Part print with two shaded views. Sizes in mm from the minimum x, y, z corner. Coordinates: 2 decimals unless noted, no trailing zeros. Write each loop counter-clockwise with the first axis right and the second up, starting at its lowest first coordinate (ties: lowest second). Pieces come first, ordered by that corner, then holes. Notation, with made-up numbers: M -23.75,29.25 L 19.25,29.25 A21 ccw 19.25,41.25 Z; hole C 53.5,-27 d7. An arc over 180 degrees is marked long. One line per question, with ' | ' between items. Start each with the question number.
(1) Flat gauge pins, fed straight in: pin 1 Ø5 at (y, z) = (7, 8) entering from -X; pin 2 Ø4.5 at (x, y) = (17.5, 17.5) entering from -Z. Where does each tip first touch, or does it go through?
(2) Two-plate mould, pull along Y, no slides. Class the marked faces 1, 2 and 3: +Y half, -Y half, draft (parallel to the pull), parting line (faces both ways), or undercut.
(3) Cut at D-D (x = 12.5). Write the cut outline in (y, z).
(4) Wall check: probe 1 along Y at (x, z) = (17.5, 2.5); probe 2 along Z at (x, y) = (4.5, 10); probe 3 along X at (y, z) = (5, 9). Give the ranges that are in metal, low to high.
(5) Cut at B-B (z = 3.5). Write the cut outline in (x, y).
(6) Cut at A-A (x = 17.5). Write the cut outline in (y, z).
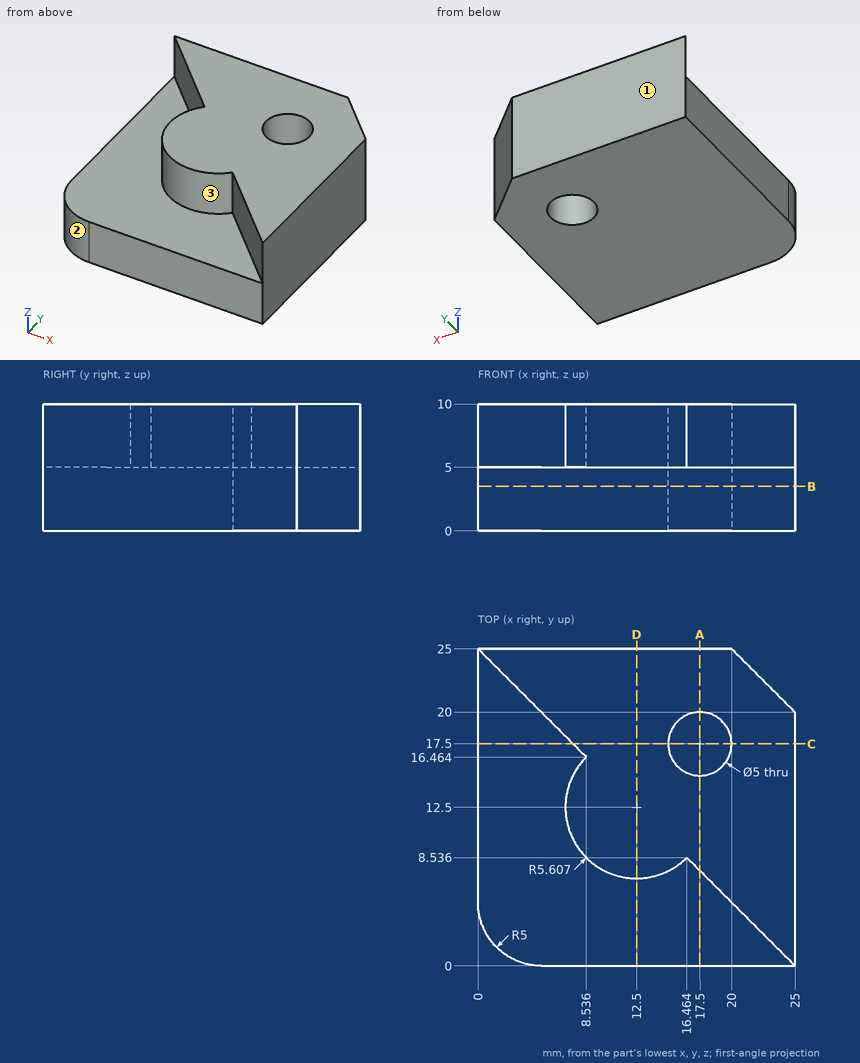
Filled in:
1) pin 1: x = 7.76 | pin 2: through
2) face 1: +Y half | face 2: -Y half | face 3: undercut
3) outline: M 0,0 L 25,0 L 25,10 L 6.89,10 L 6.89,5 L 0,5 Z
4) probe 1: 0 to 15, 20 to 25 | probe 2: 0 to 5 | probe 3: 20 to 25
5) outline: M 0,5 A5 ccw 5,0 L 25,0 L 25,20 L 20,25 L 0,25 Z; hole C 17.5,17.5 d5
6) outline: M 0,0 L 15,0 L 15,10 L 7.5,10 L 7.5,5 L 0,5 Z; M 20,0 L 25,0 L 25,10 L 20,10 Z
